from build123d import *

# Parameters (mm, degrees)
CUT_EXTRUDE1_DEPTH = 16
CIRPATTERN1_COUNT  = 24


with BuildPart() as part:
    # Sketch1 → Revolve1 (revolve)
    with BuildSketch(Plane.XY, mode=Mode.PRIVATE) as revolve1_sk:
        Polygon((-13.5, 3), (13.5, 3), (13.5, 21), (11, 21), (11, 18.45), (11, 18.2), (-5, 18.2), (-5, 18.45), (-5, 21), (-7.5, 21), (-7.5, 13), (-13.5, 13), align=None)
    revolve(revolve1_sk.sketch.rotate(Axis((-13.5, 0, 0), (1, 0, 0)), 180), axis=Axis((-13.5, 0, 0), (1, 0, 0)))

    # Sketch3 → Cut-Extrude1 (cut)
    with BuildSketch(Plane(origin=(-5, 0, 0), x_dir=(0, 0, -1), z_dir=(1, 0, 0))):
        with BuildLine():
            Line((-1.844146703, 18.106328257), (-1.35, 17.046627232))
            Line((-1.35, 17.046627232), (1.35, 17.046627232))
            Line((1.35, 17.046627232), (1.844146703, 18.106328257))
            ThreePointArc((1.844146703, 18.106328257), (0, 18.2), (-1.844146703, 18.106328257))
        make_face()
    cut_extrude1 = extrude(amount=CUT_EXTRUDE1_DEPTH, mode=Mode.SUBTRACT)

    # CirPattern1: Cut-Extrude1 ×24 about axis
    cirpattern1_axis = Axis((0, 0, 0), (1, 0, 0))
    for i in range(1, CIRPATTERN1_COUNT):
        add(cut_extrude1.rotate(cirpattern1_axis, i * 360 / CIRPATTERN1_COUNT), mode=Mode.SUBTRACT)


solid = part.part
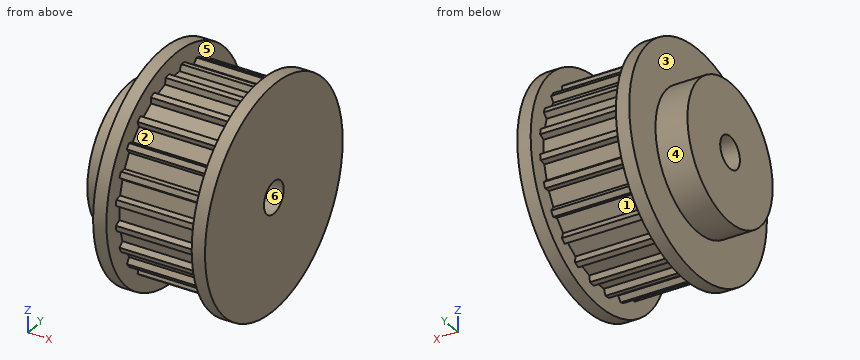
Build history of the part. All positions in model axes, mm. Face numbers are marked on the shaded views. A direction names the side the tool comes from. Round coordinates to 2 decimals unless told otherwise and drop trailing zeros. Write each loop counter-clockwise with the first axis right and the second up, starting at its lowest first coordinate (ties: lowest second). Pieces come first, ordered by that corner, then holes. Notation, with made-up numbers: M 42.25,-35 L 55.25,-35 A19 ccw 55.25,2 Z; hole C 74.25,-33.5 d11. An arc over 180 degrees is marked long. Answer as a JSON object with one key per item and string values. Group by question number.
(1) Cut at C-C (x = -9). Give the cut face in (y, z), and give its area (3 significant figures).
(2) Mould opens along Y. For the marked faces 1, 2, 3 and 4 say: pulls with the +Y half, pulls with the -Y half, needs draft (parallel to the pull), parting line crosses it, or undercut.
(3) Cut at A-A (z = 0). Give the cut face in (x, y), and give its area (3 significant figures).
(4) Which spindle directions (+Z, -Z, +X, -X, +Y, -Y) get a long thin tool onto all of the face, cutting with end or side? Do the marked faces 5 and 6. Say none if no direction does.
(5) Flat gauge pins, fed straight in: pin 1 (10 mm diameter, centred on x = -8, y = -2.5, fed in from +Z); pin 2 (1 mm diameter, centred on x = -3, y = -7, fed in from -Z); pin 3 (1.4 mm diameter, centred on x = 0.5, z = 0, fed in from -Y); pin 4 (8 mm diameter, centred on x = 10.5, z = 0, fed in from -Y). Where does each tip first touch, or does it go through?
(6) Drill centre lines: L1, parallel to Z at x = 2, y = 0; L2, parallel to X at y = 8.5, z = 15; L3, parallel to Z at x = -6, y = 0. Where is each one in solid material? Low to high.
Responses:
{
 "1": {"outline": "C 0,0 d26; hole C 0,0 d6", "area": "503 mm2"},
 "2": {"face 1": "undercut", "face 2": "undercut", "face 3": "needs draft", "face 4": "parting line crosses it"},
 "3": {"outline": "M -13.5,-13 L -7.5,-13 L -7.5,-21 L -5,-21 L -5,-17.05 L 11,-17.05 L 11,-21 L 13.5,-21 L 13.5,-3 L -13.5,-3 Z; M -13.5,3 L 13.5,3 L 13.5,21 L 11,21 L 11,17.05 L -5,17.05 L -5,21 L -7.5,21 L -7.5,13 L -13.5,13 Z", "area": "749 mm2"},
 "4": {"face 5": "none", "face 6": "+X, -X"},
 "5": {"pin 1": "stops at z = 21", "pin 2": "stops at z = -17", "pin 3": "stops at y = -17.05", "pin 4": "stops at y = -21"},
 "6": {"L1": "z = -17.05 to -3, 3 to 17.05", "L2": "x = -7.5 to -5, 11 to 13.5", "L3": "z = -21 to -3, 3 to 21"}
}
